Check sheet for the modelled part. Datum: model origin and axes. Units: mm. A direction names the side the tool comes from. Round coordinates to 2 decimals unless told otherwise and drop trailing zeros. Write each loop counter-clockwise with the first axis right and the second up, starting at its lowest first coordinate (ties: lowest second). Pieces come first, ordered by that corner, then holes. Notation, with made-up numbers: (33, 46) - (90, 46) arc R25 ccw to (90, 84) - close; hole circle Ø4 at (84, -34). An arc over 180 degrees is marked (long way). Use one line per item in the form item = value. Start each with the question number.
1) Scan lines: probe 1 along Y at (x, z) = (64, 39); probe 2 along X at (y, z) = (36, 30.5); probe 3 along Y at (x, z) = (72, 41). Record each from-to range of solid material in increasing order.
2) Set-up check for faces 5 (the face through (-4, 121, 50)), 6 (the face through (-2, 100, 38)): record each of +Z, -Z, +X, -X, +Y, -Y from which the full face is reachable in a straight line by a thin tool's end or side.
3) Section check B-B (y = 1). Record the boundary of the cut face in (x, z), then the cut area to 3 significant figures.
4) Gauge pin test, flat ends, axial feed: P1, Ø1, axis at x = -52, z = 44.5, coming from the -Y side; P2, Ø1, axis at x = 137, y = -90, coming from the +Z side. Record the tip position at first contact, or that the pin passes through.
5) Section check A-A (x = -109). Record the boundary of the cut face in (y, z).
6) Draft check along X on faces 1 (the face through (-2, 1, 25)), 2 (the face through (-4, -275, 20)), 3 (the face through (-275, -4, 20)), 4 (the face through (150, -1, 38)). Enter one of: +X half, -X half, draft (parallel to the pull), parting line (faces both ways), or undercut.
from build123d import *

# Parameters (mm, degrees)
F0_W     = 550
F0_H     = 550
F1_DEPTH = 50
F2_R     = 10
F3_W     = 300
F3_H     = 200
F4_DEPTH = 25
F5_DEPTH = 25


with BuildPart() as f1:
    # F0 (on Top) → F1 (new body)
    with BuildSketch(Plane.XY):
        Rectangle(F0_W, F0_H)
    extrude(amount=F1_DEPTH)

    # F2
    f2_edges = [f1.edges().sort_by_distance(p)[0] for p in [
        (-275, 0, 50),
        (0, 275, 50),
        (275, 0, 50),
        (0, -275, 50),
    ]]
    fillet(f2_edges, radius=F2_R)

    # F3 (on face) → F4 (join)
    with BuildSketch(Plane.XY.offset(50)):
        Rectangle(F3_W, F3_H)
    extrude(amount=-F4_DEPTH)

    # F3 (on face) → F5 (cut)
    with BuildSketch(Plane.XY.offset(50)):
        Rectangle(F3_W, F3_H)
    extrude(amount=-F5_DEPTH, mode=Mode.SUBTRACT)


solid = f1.part
Results are:
q1.probe_1 = -275 to -100, 100 to 275
q1.probe_2 = -275 to -150, 150 to 275
q1.probe_3 = -274.95 to -100, 100 to 274.95
q2.face_5 = +Z, +X, -X, +Y, -Y
q2.face_6 = +Z
q3.outline = (-275, 0) - (275, 0) - (275, 40) arc R10 ccw to (265, 50) - (150, 50) - (150, 25) - (-150, 25) - (-150, 50) - (-265, 50) arc R10 ccw to (-275, 40) - close
q3.area = 20,000 mm²
q4.P1 = -274.17
q4.P2 = 25
q5.outline = (-275, 0) - (275, 0) - (275, 40) arc R10 ccw to (265, 50) - (100, 50) - (100, 25) - (-100, 25) - (-100, 50) - (-265, 50) arc R10 ccw to (-275, 40) - close
q6.face_1 = undercut
q6.face_2 = draft
q6.face_3 = -X half
q6.face_4 = undercut
